Input: part model. Units: mm. Frame: model coordinates. A direction names the side the tool comes from. Round coordinates to 2 decimals unless told otherwise and drop trailing zeros. Write each loop counter-clockwise with the first axis right and the second up, starting at its lowest first coordinate (ties: lowest second). Pieces come first, ordered by that corner, then holes. Notation, with made-up numbers: (-32, 44.25) -> (-25, 44.25) arc R17 ccw to (-25, 57.25) -> close; hole circle Ø1 at (79.5, 34). An arc over 180 degrees is marked (long way). Write item = value, one per line.
```python
from build123d import *

# Parameters (mm, degrees)
F0_R     = 4.25
F1_DEPTH = 3
F2_R     = 15
F3_DEPTH = 6.6
F4_R     = 15
F5_DEPTH = 3
F6_DEPTH = 12.6
F7_COUNT = 30
F8_DEPTH = 25


with BuildPart() as f1:
    # F0 (on Top) → F1 (new body)
    with BuildSketch(Plane.XY):
        with BuildLine():
            ThreePointArc((0.9718013796, -14.9684869669), (10.9447937553, -10.2572652132), (15, 0))
            ThreePointArc((15, 0), (-10.2572652132, 10.9447937553), (-0.9718013796, -14.9684869669))
            ThreePointArc((-0.9718013796, -14.9684869669), (0, -15), (0.9718013796, -14.9684869669))
        make_face()
        Polygon((0, 7.5055534995), (6.5, 3.7527767497), (6.5, -3.7527767497), (0, -7.5055534995), (-6.5, -3.7527767497), (-6.5, 3.7527767497), align=None, mode=Mode.SUBTRACT)
        Polygon((6.5, -3.7527767497), (6.5, 3.7527767497), (0, 7.5055534995), (-6.5, 3.7527767497), (-6.5, -3.7527767497), (0, -7.5055534995), align=None)
        Circle(F0_R, mode=Mode.SUBTRACT)
        Circle(F0_R)
    extrude(amount=F1_DEPTH)

    # F2 (on face) → F3 (join)
    with BuildSketch(Plane.XY.offset(3)):
        Circle(F2_R)
        Polygon((-6.5, -3.7527767497), (-6.5, 3.7527767497), (0, 7.5055534995), (6.5, 3.7527767497), (6.5, -3.7527767497), (0, -7.5055534995), align=None, mode=Mode.SUBTRACT)
    extrude(amount=F3_DEPTH)

    # F4 (on face) → F5 (join)
    with BuildSketch(Plane.XY.offset(9.6)):
        Circle(F4_R)
        Polygon((6.5, -3.7527767497), (0, -7.5055534995), (-6.5, -3.7527767497), (-6.5, 3.7527767497), (0, 7.5055534995), (6.5, 3.7527767497), align=None, mode=Mode.SUBTRACT)
        Polygon((-6.5, -3.7527767497), (0, -7.5055534995), (6.5, -3.7527767497), (6.5, 3.7527767497), (0, 7.5055534995), (-6.5, 3.7527767497), align=None)
    extrude(amount=F5_DEPTH)



with BuildPart() as f6:
    # F0 (on Top) → F6 (new body, through all)
    with BuildSketch(Plane.XY):
        with BuildLine():
            ThreePointArc((0.9718013796, -14.9684869669), (0, -15), (-0.9718013796, -14.9684869669))
            ThreePointArc((-0.9718013796, -14.9684869669), (0, -15.9723121888), (0.9718013796, -14.9684869669))
        make_face()
    extrude(amount=F6_DEPTH)


with BuildPart() as f1_1:
    add(f1.part)

    add(f6.part)  # F7 merges F6
    # F7: F6 ×30 about axis
    f7_axis = Axis((0, 0, 0), (0, 0, 1))
    for i in range(1, F7_COUNT):
        add(f6.part.rotate(f7_axis, i * 360 / F7_COUNT))

    # F0 (on Top) → F8 (cut)
    with BuildSketch(Plane.XY):
        Circle(F0_R)
    extrude(amount=F8_DEPTH, mode=Mode.SUBTRACT)


solid = f1_1.part
```
1) Draft query along X for faces 1 (the face through (-10.031, 11.153, 6.212)), 2 (the face through (15, 0, 6)), 3 (the face through (4, -3, 0)). Return one class per face: +X half, -X half, draft (parallel to the pull), parting line (faces both ways), or undercut.
Solutions:
face_1 = undercut
face_2 = +X half
face_3 = draft
2) First-contact query: P1, Ø4, axis at y = -12, z = 2, coming from the -X side; P2, Ø5, axis at y = 11.5, z = 9, coming from the +X side; P3, Ø1.5, axis at y = -0.5, z = 8, coming from the +X side. Flat tips, straight axial feed; report the tip coordinate or a pass-through.
Solutions:
P1 = -12.12
P2 = 12.12
P3 = 15.84
3) Cut plane B-B (x = -1.5). Return the cut outline in (y, z).
Solutions:
outline = (-14.92, 0) -> (-3.98, 0) -> (-3.98, 3) -> (-6.64, 3) -> (-6.64, 9.6) -> (-3.98, 9.6) -> (-3.98, 12.6) -> (-14.92, 12.6) -> close; (3.98, 0) -> (14.92, 0) -> (14.92, 12.6) -> (3.98, 12.6) -> (3.98, 9.6) -> (6.64, 9.6) -> (6.64, 3) -> (3.98, 3) -> close
4) Access query for faces 4 (the face through (-9.406, -12.909, 6.212)), 5 (the face through (-1.576, -14.917, 6.212)), 6 (the face through (-6.5, 0, 6)). Directions: +Z, -Z, +X, -X, +Y, -Y. A direction counts if a zero-diameter tool reaches every point of the face in a straight line with its end or side. Return the directions, or none.
Solutions:
face_4 = +Z, -Z
face_5 = +Z, -Z, -Y
face_6 = none
5) Cut plane A-A (y = -2). Return the cut outline in (x, z), and give its area (3 significant figures).
Solutions:
outline = (-15.79, 0) -> (-3.75, 0) -> (-3.75, 3) -> (-6.5, 3) -> (-6.5, 9.6) -> (-3.75, 9.6) -> (-3.75, 12.6) -> (-15.79, 12.6) -> close; (3.75, 0) -> (15.79, 0) -> (15.79, 12.6) -> (3.75, 12.6) -> (3.75, 9.6) -> (6.5, 9.6) -> (6.5, 3) -> (3.75, 3) -> close
area = 267 mm^2
6) Line query: L1, parallel to X at y = 0, z = 11.5; L2, parallel to Y at x = 0, z = 1.7; L3, parallel to Y at x = 12, z = 9.25. Output: solid intervals per line, ascending. Write a range as from..to.
Solutions:
L1 = -15..-4.25, 4.25..15
L2 = -15.97..-4.25, 4.25..15.97
L3 = -10.5..-9.57, -9..9, 9.57..10.5
